The listing builds one solid part. Answer for the finished solid, in the listing's coordinates (mm). A direction names the side the tool comes from. Round coordinates to 2 decimals unless told otherwise and drop trailing zeros. Order: outer loops, then holes, each group sorted by start corner. A loop starts at its lowest first (then second) coordinate and runs counter-clockwise, first axis right, second up. Notation, with made-up numbers: (-32.5, -32.75) - (9.5, -32.75) arc R35 cw to (9.5, 4.25) - close; hole circle Ø2 at (74.5, 32.5). An arc over 180 degrees is marked (long way). Use CSV: the item, a comma, the result in double quotes. Start each with the question number.
Item 1: Flat-ended cylindrical pins translate along their axes: P1, Ø2, axis at x = 89.5, z = -64, coming from the +Y side; P2, Ø2, axis at y = -48, z = -63, coming from the -X side; P3, Ø5.5, axis at x = 89, z = -38.5, coming from the +Y side; P4, Ø3.5, axis at x = 90, z = -40, coming from the +Y side (1 decimal). Find the tip coordinate at first contact, or state that the pin passes through.
Item 2: Find section A-A, the plane z = -62.5. Give the vertices of the cut face in (x, y).
Item 3: Determine the mould class of faces 3 (the flat face through (56, -54, -36)), 4 (the flat face through (92.764, -47.262, -37.859)) for opening direction X: +X half, -X half, draft (parallel to the pull), parting line (faces both ways), or undercut.
Item 4: Find section B-B, the plane z = -54. Give the vertices of the cut face in (x, y).
Item 5: For faces 1 (the flat face through (88.292, -44.722, -59.486)), 2 (the flat face through (66, -39, -72.5)), determine the directions among +Z, -Z, +X, -X, +Y, -Y from which every point of the face is accessible in a straight line to the end or side of a thin tool.
Item 6: Find section D-D, the plane x = 82. Give the vertices of the cut face in (y, z), plus the area to 3 significant figures.
Item 7: Straight lines are drawn through the part: line 1 along Z through (x, y) = (90, -52.45); line 2 along Y through (x, z) = (93.5, -40); line 3 along Y through (x, z) = (38, -47.5). For each, find the intervals that lie inside material, in ascending order. Write a range as [from, to].
Item 8: Find section C-C, the plane y = -29.5. Give the vertices of the cut face in (x, z).
```python
from build123d import *

# Parameters (mm, degrees)
EXTRUDE_1_DEPTH     = 72.5
FILLET_1_R          = 0.5
CUT_EXTRUDE_1_DEPTH = 49
SKETCH_5_R          = 2.05
CUT_EXTRUDE_2_DEPTH = 5
SKETCH_6_R          = 74.194648386
CUT_EXTRUDE_3_DEPTH = 135.804488056


with BuildPart() as part:
    # 草图3 → 凸台-拉伸1 (new, symmetric)
    with BuildSketch(Plane.XY):
        with BuildLine():
            Line((100, -54), (0, -54))
            ThreePointArc((0, -54), (38.183766184, -38.183766184), (54, 0))
            Line((54, 0), (100, -54))
        make_face()
    extrude(amount=EXTRUDE_1_DEPTH, both=True)

    # 圆角1
    fillet_1_edges = [part.edges().sort_by_distance(p)[0] for p in [
        (54, 0, 0),
        (0, -54, 0),
    ]]
    fillet(fillet_1_edges, radius=FILLET_1_R)

    # 草图4 → 切除-拉伸1 (cut)
    with BuildSketch(Plane(origin=(0, 0, 0), x_dir=(1, 0, 0), z_dir=(0, 1, 0))):
        Polygon((93.464101615, -64.5), (93.464101615, -60.5), (90, -58.5), (86.535898385, -60.5), (86.535898385, -64.5), (90, -66.5), align=None)
        Polygon((29.892304845, -58.5), (26.42820323, -60.5), (26.42820323, -64.5), (29.892304845, -66.5), (33.356406461, -64.5), (33.356406461, -60.5), align=None)
        Polygon((33.356406461, 60.5), (29.892304845, 58.5), (26.42820323, 60.5), (26.42820323, 64.5), (29.892304845, 66.5), (33.356406461, 64.5), align=None)
        Polygon((90, 66.5), (93.464101615, 64.5), (93.464101615, 60.5), (90, 58.5), (86.535898385, 60.5), (86.535898385, 64.5), align=None)
        Polygon((92, -36.535898385), (88, -36.535898385), (86, -40), (88, -43.464101615), (92, -43.464101615), (94, -40), align=None)
        Polygon((94, 40), (92, 43.464101615), (88, 43.464101615), (86, 40), (88, 36.535898385), (92, 36.535898385), align=None)
    extrude(amount=-CUT_EXTRUDE_1_DEPTH, mode=Mode.SUBTRACT)

    # 草图5 → 切除-拉伸2 (cut)
    with BuildSketch(Plane(origin=(0, -49, 0), x_dir=(1, 0, 0), z_dir=(0, 1, 0))):
        with Locations(Location((29.892304845, -62.5, 0), (0, 0, 180))):
            Circle(SKETCH_5_R)
        with Locations((29.892304845, 62.5)):
            Circle(SKETCH_5_R)
        with Locations(Location((90, 62.5, 0), (0, 0, 180))):
            Circle(SKETCH_5_R)
        with Locations((90, -62.5)):
            Circle(SKETCH_5_R)
        with Locations(Location((90, 40, 0), (0, 0, 180))):
            Circle(SKETCH_5_R)
        with Locations(Location((90, -40.064560571, 0), (0, 0, 180))):
            Circle(SKETCH_5_R)
    extrude(amount=-CUT_EXTRUDE_2_DEPTH, mode=Mode.SUBTRACT)

    # 草图6 → 切除-拉伸3 (cut, through all)
    with BuildSketch(Plane.XY):
        with Locations((51.898746265, -54)):
            Circle(SKETCH_6_R)
    extrude(amount=CUT_EXTRUDE_3_DEPTH, mode=Mode.SUBTRACT)


solid = part.part
```
Worked out:
1,P1,"stops at y = -49"
1,P2,"stops at x = 22.69"
1,P3,"stops at y = -37.86"
1,P4,"passes through"
2,outline,"(10.3, -53.01) arc R0.5 ccw to (10.39, -54) - (27.84, -54) - (27.84, -49) - (26.43, -49) - (26.43, -47.09) arc R54 cw to start; (31.94, -54) - (87.95, -54) - (87.95, -49) - (86.54, -49) - (86.54, -38.19) - (54.86, -1.01) arc R0.5 ccw to (53.98, -1.33) arc R54 cw to (33.36, -42.47) - (33.36, -49) - (31.94, -49) - close; (92.05, -54) - (100, -54) - (93.46, -46.33) - (93.46, -49) - (92.05, -49) - close"
3,face 3,"draft"
3,face 4,"undercut"
4,outline,"(10.3, -53.01) arc R0.5 ccw to (10.39, -54) - (100, -54) - (54.86, -1.01) arc R0.5 ccw to (53.98, -1.33) arc R54 cw to start"
5,face 1,"+Y"
5,face 2,"-Z, +X, -X, +Y, -Y"
6,outline,"(-54, -72.5) - (-32.87, -72.5) - (-32.87, 0) - (-54, 0) - close"
6,area,"1,530 mm²"
7,line 1,"z = [-72.5, -64.55], [-60.45, -42.05], [-37.95, 0]"
7,line 2,"y = [-54, -49]"
7,line 3,"y = [-54, -38.37]"
8,outline,"(45.23, -72.5) - (79.13, -72.5) - (79.13, 0) - (45.23, 0) - close"
